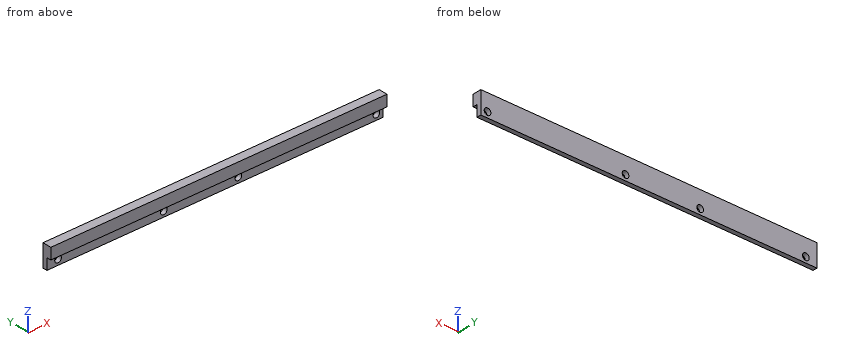
```python
from build123d import *

# Parameters (mm, degrees)
SKETCH_1_W      = 151
SKETCH_1_H      = 5
SKETCH_1_R      = 1.5
EXTRUDE_1_DEPTH = 2
EXTRUDE_START   = 2
SKETCH_2_W      = 151
SKETCH_2_H      = 5
EXTRUDE_2_DEPTH = 4


with BuildPart() as part:
    # 草图1 → 凸台-拉伸1 (new body)
    with BuildSketch(Plane(origin=(0, 0, 0), x_dir=(1, 0, 0), z_dir=(0, 1, 0))):
        with Locations((75.5, -2.5)):
            Rectangle(SKETCH_1_W, SKETCH_1_H)
        with Locations(Location((5, -2.5, 0), (0, 0, 270))):
            Circle(SKETCH_1_R, mode=Mode.SUBTRACT)
        with Locations(Location((52.5, -2.5, 0), (0, 0, 270))):
            Circle(SKETCH_1_R, mode=Mode.SUBTRACT)
        with Locations(Location((86, -2.5, 0), (0, 0, 270))):
            Circle(SKETCH_1_R, mode=Mode.SUBTRACT)
        with Locations(Location((148, -2.5, 0), (0, 0, 270))):
            Circle(SKETCH_1_R, mode=Mode.SUBTRACT)
    extrude(amount=EXTRUDE_1_DEPTH)

    # 草图2 → 凸台-拉伸2 (add)
    with BuildSketch(Plane(origin=(0, 0, 0), x_dir=(1, 0, 0), z_dir=(0, 1, 0)).offset(EXTRUDE_START)):
        with Locations((75.5, -7.5)):
            Rectangle(SKETCH_2_W, SKETCH_2_H)
    extrude(amount=-EXTRUDE_2_DEPTH)


solid = part.part
```
Work out the finished part from the listing and answer in its coordinate system (mm). Round coordinates to 2 decimals unless told otherwise and drop trailing zeros. Write each loop counter-clockwise with the first axis right and the second up, starting at its lowest first coordinate (ties: lowest second). Pieces come first, ordered by that corner, then holes.
1) A cutting plane is placed at B-B on x = 148. Determine the outline of the cut face in (y, z), and give its area (3 significant figures).
2) A cutting plane is placed at D-D on y = -1.15. Determine the outline of the cut face in (x, z).
3) Flat-ended cylindrical pins translate along their axes: P1, Ø4, axis at x = 148, z = 2.5, coming from the +Y side; P2, Ø1.6, axis at x = 38.5, y = -1.5, coming from the -Z side; P3, Ø4, axis at x = 5, z = 2.5, coming from the -Y side. Find the tip coordinate at first contact, or state that the pin passes through.
4) A cutting plane is placed at C-C on x = 11. Determine the outline of the cut face in (y, z).
5) Consider probe 1 along X at (y, z) = (1.5, 2.5); probe 2 along X at (y, z) = (1.2, 1.5); probe 3 along Y at (x, z) = (41.5, 2.5). Determine where each line is inside the solid, lowest interval first.
6) A cutting plane is placed at A-A on z = 2.5. Determine the outline of the cut face in (x, y).
Entries:
1. outline: (-2, 5) - (0, 5) - (0, 4) - (2, 4) - (2, 10) - (-2, 10) - close; (0, 0) - (2, 0) - (2, 1) - (0, 1) - close
1. area: 24.0 mm2
2. outline: (0, 5) - (151, 5) - (151, 10) - (0, 10) - close
3. P1: stops at y = 2
3. P2: stops at z = 5
3. P3: stops at y = 0
4. outline: (-2, 5) - (0, 5) - (0, 0) - (2, 0) - (2, 10) - (-2, 10) - close
5. probe 1: x = 0 to 3.5, 6.5 to 51, 54 to 84.5, 87.5 to 146.5, 149.5 to 151
5. probe 2: x = 0 to 3.88, 6.12 to 51.38, 53.62 to 84.88, 87.12 to 146.88, 149.12 to 151
5. probe 3: y = 0 to 2
6. outline: (0, 0) - (3.5, 0) - (3.5, 2) - (0, 2) - close; (6.5, 0) - (51, 0) - (51, 2) - (6.5, 2) - close; (54, 0) - (84.5, 0) - (84.5, 2) - (54, 2) - close; (87.5, 0) - (146.5, 0) - (146.5, 2) - (87.5, 2) - close; (149.5, 0) - (151, 0) - (151, 2) - (149.5, 2) - close
